Can you work these out from the model? Positions are in its coordinate system, mm. A direction names the side the tool comes from. Give positions to 0.01 mm unless a question says otherwise; leave off trailing zeros. Loops run counter-clockwise (first coordinate to the right, second up) from the corner with the lowest first, then second, coordinate; pieces in that order, holes last. Notation, with made-up numbers: (-8.75, -9.5) - (5.25, -9.5) arc R14 cw to (5.25, 17.5) - close; hole circle Ø5 at (41, 82). An arc over 180 degrees is marked (long way). Answer as a JSON object with one key per item and string values.
```python
from build123d import *

# Parameters (mm, degrees)
F0_R     = 9.525
F1_DEPTH = 2.54
F2_R     = 1.7145
F3_DEPTH = 25.4
F4_R     = 2.53999


# Not quite as in the source:
# - a fillet or chamfer is up to 0.001 mm smaller than in the source, because OpenCascade refuses the exact size


with BuildPart() as f1:
    # F0 (on Top) → F1 (new body)
    with BuildSketch(Plane.XY):
        Circle(F0_R)
    extrude(amount=F1_DEPTH)

    # F2 (on face) → F3 (join)
    with BuildSketch(Plane.XY.offset(2.54)):
        with BuildLine():
            ThreePointArc((9.525, 0), (9.4767668574, 0.9573478631), (9.33255592, 1.905))
            ThreePointArc((9.33255592, 1.905), (7.5646235439, 0), (9.33255592, -1.905))
            ThreePointArc((9.33255592, -1.905), (9.4767668574, -0.9573478631), (9.525, 0))
        make_face()
        with BuildLine():
            ThreePointArc((-1.905, 9.33255592), (0, 7.5646235439), (1.905, 9.33255592))
            ThreePointArc((1.905, 9.33255592), (0, 9.525), (-1.905, 9.33255592))
        make_face()
        with BuildLine():
            ThreePointArc((-9.33255592, -1.905), (-7.5646235439, 0), (-9.33255592, 1.905))
            ThreePointArc((-9.33255592, 1.905), (-9.525, 0), (-9.33255592, -1.905))
        make_face()
        with BuildLine():
            ThreePointArc((-1.905, -9.33255592), (0, -9.525), (1.905, -9.33255592))
            ThreePointArc((1.905, -9.33255592), (0, -7.5646235439), (-1.905, -9.33255592))
        make_face()
        Circle(F2_R)
    extrude(amount=F3_DEPTH)

    # F4 (radius 2.54 in the source; OpenCascade refuses exactly that, so slightly less here)
    f4_edges = [f1.edges().sort_by_distance(p)[0] for p in [
        (-9.525, 0, 0),
    ]]
    fillet(f4_edges, radius=F4_R)


solid = f1.part
```
1) Which directions (+Z, -Z, +X, -X, +Y, -Y) give clear straight access to the entire face, cutting with the end or side of a thin tool? Please do faces 1 (the flat face through (9, 0, 27.94)), 2 (the cylindrical face through (-7.565, -0.04, 15.062)).
Check sheet entries:
{"face 1": "+Z, +X, -X, +Y, -Y", "face 2": "+Z"}
2) Imagine slicing it at B-B on x = 0. Write out the boundary of the cut face in (y, z) (1 decimal), and give its area (3 significant figures).
Check sheet entries:
{"outline": "(-9.5, 2.5) arc R2.5 ccw to (-7, 0) - (7, 0) arc R2.5 ccw to (9.5, 2.5) - (9.5, 27.9) - (7.6, 27.9) - (7.6, 2.5) - (1.7, 2.5) - (1.7, 27.9) - (-1.7, 27.9) - (-1.7, 2.5) - (-7.6, 2.5) - (-7.6, 27.9) - (-9.5, 27.9) - close", "area": "232 mm2"}
3) I need wall thicknesses on L1, parallel to X at y = 0.75, z = 7.75; L2, parallel to X at y = 1.5, z = 24.75; L3, parallel to Y at x = 0.25, z = 15. Which ranges of each line are inside material? Lowest first, please.
Check sheet entries:
{"L1": "-9.5 to -7.72, -1.54 to 1.54, 7.72 to 9.5", "L2": "-9.41 to -8.29, -0.83 to 0.83, 8.29 to 9.41", "L3": "-9.52 to -7.58, -1.7 to 1.7, 7.58 to 9.52"}
4) If we mould it in two halves opening along X, with no side actions, what happens to faces 3 (the cylindrical face through (-0.372, -1.674, 15.062)), 4 (the flat face through (0, 0, 27.94)), 5 (the cylindrical face through (0.04, -7.565, 15.062))? For each: released by +X, released by -X, zero draft, split by the parting line, or undercut.
Check sheet entries:
{"face 3": "undercut", "face 4": "zero draft", "face 5": "split by the parting line"}
5) I'm going to push flat-ended pins straight in: P1, Ø6, axis at x = 4.5, z = 7, coming from the +Y side; P2, Ø2, axis at y = 1.5, z = 8.5, coming from the +X side. Where does each tip first touch, or does it pass through?
Check sheet entries:
{"P1": "y = 9.41", "P2": "x = 9.51"}
6) Imagine slicing it at A-A on z = 13. Give the number of separate pieces and of enclosed holes in the cut face, and give its area (3 significant figures).
Check sheet entries:
{"separate pieces": "5", "enclosed holes": "0", "area": "31.9 mm2"}
